The figure shows three views and two pictorial views of one solid part (mm, origin at its lowest corner). Answer the questions. Coordinates: 2 decimals unless noted, no trailing zeros. Order: outer loops, then holes, each group sorted by start corner. A loop starts at its lowest first (then second) coordinate and runs counter-clockwise, first axis right, second up.
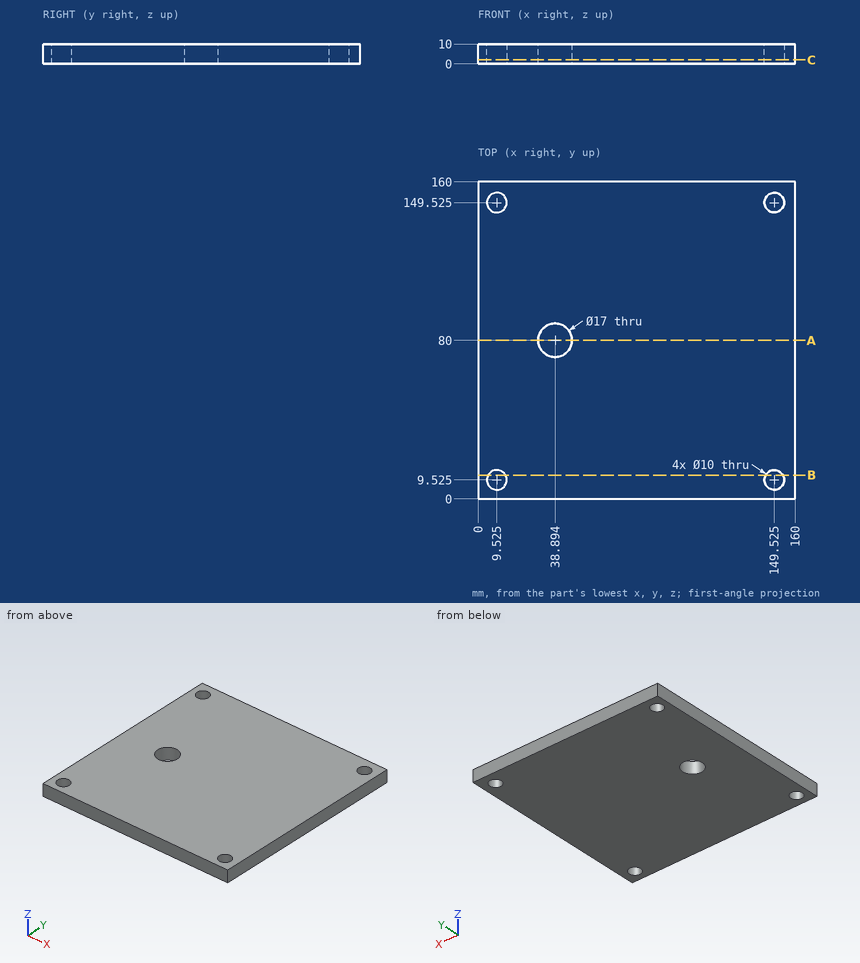
1) Straight lines are drawn through the part: probe 1 along X at (y, z) = (80, 5.25); probe 2 along Y at (x, z) = (32, 4.5); probe 3 along X at (y, z) = (84.5, 8.25) (1 decimal). For each, find the intervals that lie inside material, in ascending order.
2) A cutting plane is placed at C-C, the plane z = 2. Write down the section's boundary in (x, y) (1 decimal).
3) A cutting plane is placed at B-B, the plane y = 12. Write down the section's boundary in (x, z), plus the area to 3 significant figures.
4) A cutting plane is placed at A-A, the plane y = 80. Write down the section's boundary in (x, z), plus the area to 3 significant figures.
Working result:
1. probe 1: x = 0 to 30.39, 47.39 to 160
1. probe 2: y = 0 to 75.03, 84.97 to 160
1. probe 3: x = 0 to 31.7, 46.1 to 160
2. outline: (0, 0) - (160, 0) - (160, 160) - (0, 160) - close; hole circle Ø10 at (9.5, 9.5); hole circle Ø10 at (9.5, 149.5); hole circle Ø17 at (38.9, 80); hole circle Ø10 at (149.5, 9.5); hole circle Ø10 at (149.5, 149.5)
3. outline: (0, 0) - (5.18, 0) - (5.18, 10) - (0, 10) - close; (13.87, 0) - (145.18, 0) - (145.18, 10) - (13.87, 10) - close; (153.87, 0) - (160, 0) - (160, 10) - (153.87, 10) - close
3. area: 1,430 mm2
4. outline: (0, 0) - (30.39, 0) - (30.39, 10) - (0, 10) - close; (47.39, 0) - (160, 0) - (160, 10) - (47.39, 10) - close
4. area: 1,430 mm2
